The model under review builds one solid part; all positions refer to its coordinate system, in mm. A direction names the side the tool comes from. Give positions to 0.01 mm unless a question says otherwise; leave off trailing zeros. Order: outer loops, then holes, each group sorted by start corner. A loop starts at its lowest first (then second) coordinate and runs counter-clockwise, first axis right, second up. Notation, with made-up numbers: (61, -31.75) -> (69, -31.75) arc R9 cw to (69, -24.75) -> close; hole circle Ø9 at (64.5, 51). An arc over 180 degrees is marked (long way). Use one line per item in the form item = value.
```python
from build123d import *

# Parameters (mm, degrees)
SKETCH1_R           = 11
BOSS_EXTRUDE1_DEPTH = 35
SKETCH2_W           = 60
SKETCH2_H           = 58
CUT_EXTRUDE1_DEPTH  = 109.857705285
CUT_EXTRUDE2_REACH  = 148.458
SKETCH3_W           = 38
SKETCH3_H           = 58


with BuildPart() as part:
    # Sketch1 → Boss-Extrude1 (new, symmetric)
    with BuildSketch(Plane(origin=(0, 0, 0), x_dir=(1, 0, 0), z_dir=(0, 1, 0))):
        with BuildLine():
            Line((-75, 25), (75, 25))
            ThreePointArc((75, 25), (100, 0), (75, -25))
            Line((75, -25), (-75, -25))
            ThreePointArc((-75, -25), (-100, 0), (-75, 25))
        make_face()
        with Locations(Location((75, 0, 0), (0, 0, 270))):
            Circle(SKETCH1_R, mode=Mode.SUBTRACT)
        with Locations(Location((-75, 0, 0), (0, 0, 270))):
            Circle(SKETCH1_R, mode=Mode.SUBTRACT)
    extrude(amount=BOSS_EXTRUDE1_DEPTH, both=True)

    # Sketch2 → Cut-Extrude1 (cut, symmetric)
    with BuildSketch(Plane.XY):
        with Locations((70, 0)):
            Rectangle(SKETCH2_W, SKETCH2_H)
    cut_extrude1 = extrude(amount=CUT_EXTRUDE1_DEPTH, both=True, mode=Mode.SUBTRACT)

    # Mirror1: Cut-Extrude1 across plane
    add(cut_extrude1.mirror(Plane(origin=(0, 0, 0), x_dir=(0, 0, 1), z_dir=(1, 0, 0))), mode=Mode.SUBTRACT)

    # Sketch3 → Cut-Extrude2 (cut, up to next)
    with BuildSketch(Plane(origin=(40, 0, 0), x_dir=(0, 0, -1), z_dir=(1, 0, 0)), mode=Mode.PRIVATE) as cut_extrude2_sk1:
        Rectangle(SKETCH3_W, SKETCH3_H)
    cut_extrude2_tool1 = extrude(cut_extrude2_sk1.sketch, amount=-CUT_EXTRUDE2_REACH, mode=Mode.PRIVATE) & part.part
    add(cut_extrude2_tool1.solids().sort_by_distance((40, 0, 0))[0], mode=Mode.SUBTRACT)


solid = part.part
```
1. Add section A-A on x = -31. Give the boundary of the cut face in (y, z), then the cut area to 3 significant figures.
Values:
outline = (-35, -25) -> (35, -25) -> (35, 25) -> (-35, 25) -> close; hole (-29, -19) -> (29, -19) -> (29, 19) -> (-29, 19) -> close
area = 1,300 mm^2
2. The part is to be moulded in two halves that separate along X. For faces 1 (the face through (85.906, 31.958, -1.432)), 2 (the face through (1, 0, -19)), 3 (the face through (-40, 0, 22)), say which applies: +X half, -X half, draft (parallel to the pull), parting line (faces both ways), or undercut.
Values:
face_1 = undercut
face_2 = draft
face_3 = -X half
3. Add section C-C on x = -51. Give the boundary of the cut face in (y, z), then the cut area to 3 significant figures.
Values:
outline = (-35, -25) -> (-29, -25) -> (-29, 25) -> (-35, 25) -> close; (29, -25) -> (35, -25) -> (35, 25) -> (29, 25) -> close
area = 600 mm^2
4. Add section D-D on y = -31. Give the boundary of the cut face in (x, z).
Values:
outline = (-75, -25) -> (75, -25) arc R25 ccw to (75, 25) -> (-75, 25) arc R25 ccw to start; hole circle Ø22 at (-75, 0); hole circle Ø22 at (75, 0)
5. For L1, parallel to X at y = 32, z = 0; L2, parallel to Z at x = -31, y = -1; L3, parallel to Z at x = 75, y = -32, list the stretches that pass through material, from the lowest coordinate up.
Values:
L1 = -100 to -86, -64 to 64, 86 to 100
L2 = -25 to -19, 19 to 25
L3 = -25 to -11, 11 to 25
6. For pin 1 Ø17.5 at (x, z) = (75, 0) entering from -Y; pin 2 Ø3 at (y, z) = (8.5, -23) entering from +X; pin 3 Ø6.5 at (y, z) = (-5, 22.5) entering from -X, all flat-tipped, find the tip position at first contact; note any pin that passes through.
Values:
pin_1 = through
pin_2 = 40
pin_3 = -40
7. Add section B-B on y = -9. Give the boundary of the cut face in (x, z), then the cut area to 3 significant figures.
Values:
outline = (-40, -25) -> (40, -25) -> (40, -19) -> (-40, -19) -> close; (-40, 19) -> (40, 19) -> (40, 25) -> (-40, 25) -> close
area = 960 mm^2
8. Tool access review of faces 4 (the face through (1, 0, 19)), 5 (the face through (40, 0, -22)), 6 (the face through (-40, 0, -22)): name each direction out of +Z, -Z, +X, -X, +Y, -Y from which nothing blocks a thin tool from reaching the whole face with its end or side.
Values:
face_4 = +X, -X
face_5 = +Z, -Z, +X
face_6 = +Z, -Z, -X
